from build123d import *

# Parameters (mm, degrees)
SALIENTE_EXTRUIR3_DEPTH = 0.02
SALIENTE_EXTRUIR5_START = -2
SALIENTE_EXTRUIR5_DEPTH = 2
CROQUIS4_R              = 0.025
SALIENTE_EXTRUIR6_DEPTH = 30
SALIENTE_EXTRUIR7_START = 0.01
CROQUIS4_2_R            = 0.025
SALIENTE_EXTRUIR7_DEPTH = 0.01


with BuildPart() as part:
    # Croquis1 → Saliente-Extruir3 (new body)
    with BuildSketch(Plane.XY):
        with BuildLine():
            Line((-0.821642524, 0), (-1.5, 0))
            ThreePointArc((-1.5, 0), (-1.803592236, -0.268799536), (-2.059736596, -0.583142508))
            Line((-2.059736596, -0.583142508), (-0.821642524, -0.583142508))
            Line((-0.821642524, -0.583142508), (0.708153247, -0.583142508))
            ThreePointArc((0.708153247, -0.583142508), (0.792032388, -0.667021649), (0.708153247, -0.75090079))
            Line((0.708153247, -0.75090079), (-0.821642524, -0.75090079))
            ThreePointArc((-0.821642524, -0.75090079), (-1.266985163, -1.19624343), (-0.821642524, -1.641586069))
            Line((-0.821642524, -1.641586069), (0.708153247, -1.641586069))
            ThreePointArc((0.708153247, -1.641586069), (0.788738621, -1.722171443), (0.708153247, -1.802756818))
            Line((0.708153247, -1.802756818), (-0.821642524, -1.802756818))
            ThreePointArc((-0.821642524, -1.802756818), (-1.277929981, -2.259044275), (-0.821642524, -2.715331733))
            Line((-0.821642524, -2.715331733), (0.708153247, -2.715331733))
            ThreePointArc((0.708153247, -2.715331733), (0.785471646, -2.792650132), (0.708153247, -2.869968532))
            Line((0.708153247, -2.869968532), (-0.821642524, -2.869968532))
            ThreePointArc((-0.821642524, -2.869968532), (-1.276795627, -3.325121635), (-0.821642524, -3.780274738))
            Line((-0.821642524, -3.780274738), (0.764779262, -3.780274738))
            Line((0.764779262, -3.780274738), (0.764779262, -4))
            Line((0.764779262, -4), (1.5, -4))
            ThreePointArc((1.5, -4), (1.806680275, -3.727977542), (2.064782817, -3.409493497))
            Line((2.064782817, -3.409493497), (-0.821642524, -3.409493497))
            ThreePointArc((-0.821642524, -3.409493497), (-0.907365435, -3.323770586), (-0.821642524, -3.238047675))
            Line((-0.821642524, -3.238047675), (0.708153247, -3.238047675))
            ThreePointArc((0.708153247, -3.238047675), (1.160084738, -2.786116183), (0.708153247, -2.334184692))
            Line((0.708153247, -2.334184692), (-0.821642524, -2.334184692))
            ThreePointArc((-0.821642524, -2.334184692), (-0.894604957, -2.261222258), (-0.821642524, -2.188259825))
            Line((-0.821642524, -2.188259825), (0.708153247, -2.188259825))
            ThreePointArc((0.708153247, -2.188259825), (1.169203972, -1.727209099), (0.708153247, -1.266158374))
            Line((0.708153247, -1.266158374), (-0.821642524, -1.266158374))
            ThreePointArc((-0.821642524, -1.266158374), (-0.890869473, -1.196931424), (-0.821642524, -1.127704475))
            Line((-0.821642524, -1.127704475), (0.708153247, -1.127704475))
            ThreePointArc((0.708153247, -1.127704475), (1.166166615, -0.669691107), (0.708153247, -0.211677738))
            Line((0.708153247, -0.211677738), (-0.821642524, -0.211677738))
            Line((-0.821642524, -0.211677738), (-0.821642524, 0))
        make_face()
    extrude(amount=SALIENTE_EXTRUIR3_DEPTH)

    # Croquis1_5 → Saliente-Extruir5 (add)
    with BuildSketch(Plane.XY.offset(SALIENTE_EXTRUIR5_START)):
        with BuildLine():
            Line((-0.821642524, -0.583142508), (-2.059736596, -0.583142508))
            ThreePointArc((-2.059736596, -0.583142508), (-2.467115713, -2.404153511), (-1.5, -4))
            Line((-1.5, -4), (0.764779262, -4))
            Line((0.764779262, -4), (0.764779262, -3.780274738))
            Line((0.764779262, -3.780274738), (-0.821642524, -3.780274738))
            ThreePointArc((-0.821642524, -3.780274738), (-1.276795627, -3.325121635), (-0.821642524, -2.869968532))
            Line((-0.821642524, -2.869968532), (0.708153247, -2.869968532))
            ThreePointArc((0.708153247, -2.869968532), (0.785471646, -2.792650132), (0.708153247, -2.715331733))
            Line((0.708153247, -2.715331733), (-0.821642524, -2.715331733))
            ThreePointArc((-0.821642524, -2.715331733), (-1.277929981, -2.259044275), (-0.821642524, -1.802756818))
            Line((-0.821642524, -1.802756818), (0.708153247, -1.802756818))
            ThreePointArc((0.708153247, -1.802756818), (0.788738621, -1.722171443), (0.708153247, -1.641586069))
            Line((0.708153247, -1.641586069), (-0.821642524, -1.641586069))
            ThreePointArc((-0.821642524, -1.641586069), (-1.266985163, -1.19624343), (-0.821642524, -0.75090079))
            Line((-0.821642524, -0.75090079), (0.708153247, -0.75090079))
            ThreePointArc((0.708153247, -0.75090079), (0.792032388, -0.667021649), (0.708153247, -0.583142508))
            Line((0.708153247, -0.583142508), (-0.821642524, -0.583142508))
        make_face()
        with BuildLine():
            Line((1.5, 0), (-0.821642524, 0))
            Line((-0.821642524, 0), (-0.821642524, -0.211677738))
            Line((-0.821642524, -0.211677738), (0.708153247, -0.211677738))
            ThreePointArc((0.708153247, -0.211677738), (1.166166615, -0.669691107), (0.708153247, -1.127704475))
            Line((0.708153247, -1.127704475), (-0.821642524, -1.127704475))
            ThreePointArc((-0.821642524, -1.127704475), (-0.890869473, -1.196931424), (-0.821642524, -1.266158374))
            Line((-0.821642524, -1.266158374), (0.708153247, -1.266158374))
            ThreePointArc((0.708153247, -1.266158374), (1.169203972, -1.727209099), (0.708153247, -2.188259825))
            Line((0.708153247, -2.188259825), (-0.821642524, -2.188259825))
            ThreePointArc((-0.821642524, -2.188259825), (-0.894604957, -2.261222258), (-0.821642524, -2.334184692))
            Line((-0.821642524, -2.334184692), (0.708153247, -2.334184692))
            ThreePointArc((0.708153247, -2.334184692), (1.160084738, -2.786116183), (0.708153247, -3.238047675))
            Line((0.708153247, -3.238047675), (-0.821642524, -3.238047675))
            ThreePointArc((-0.821642524, -3.238047675), (-0.907365435, -3.323770586), (-0.821642524, -3.409493497))
            Line((-0.821642524, -3.409493497), (2.064782817, -3.409493497))
            ThreePointArc((2.064782817, -3.409493497), (2.466390198, -1.591442305), (1.5, 0))
        make_face()
        with BuildLine():
            Line((-0.821642524, 0), (-1.5, 0))
            ThreePointArc((-1.5, 0), (-1.803592236, -0.268799536), (-2.059736596, -0.583142508))
            Line((-2.059736596, -0.583142508), (-0.821642524, -0.583142508))
            Line((-0.821642524, -0.583142508), (0.708153247, -0.583142508))
            ThreePointArc((0.708153247, -0.583142508), (0.792032388, -0.667021649), (0.708153247, -0.75090079))
            Line((0.708153247, -0.75090079), (-0.821642524, -0.75090079))
            ThreePointArc((-0.821642524, -0.75090079), (-1.266985163, -1.19624343), (-0.821642524, -1.641586069))
            Line((-0.821642524, -1.641586069), (0.708153247, -1.641586069))
            ThreePointArc((0.708153247, -1.641586069), (0.788738621, -1.722171443), (0.708153247, -1.802756818))
            Line((0.708153247, -1.802756818), (-0.821642524, -1.802756818))
            ThreePointArc((-0.821642524, -1.802756818), (-1.277929981, -2.259044275), (-0.821642524, -2.715331733))
            Line((-0.821642524, -2.715331733), (0.708153247, -2.715331733))
            ThreePointArc((0.708153247, -2.715331733), (0.785471646, -2.792650132), (0.708153247, -2.869968532))
            Line((0.708153247, -2.869968532), (-0.821642524, -2.869968532))
            ThreePointArc((-0.821642524, -2.869968532), (-1.276795627, -3.325121635), (-0.821642524, -3.780274738))
            Line((-0.821642524, -3.780274738), (0.764779262, -3.780274738))
            Line((0.764779262, -3.780274738), (0.764779262, -4))
            Line((0.764779262, -4), (1.5, -4))
            ThreePointArc((1.5, -4), (1.806680275, -3.727977542), (2.064782817, -3.409493497))
            Line((2.064782817, -3.409493497), (-0.821642524, -3.409493497))
            ThreePointArc((-0.821642524, -3.409493497), (-0.907365435, -3.323770586), (-0.821642524, -3.238047675))
            Line((-0.821642524, -3.238047675), (0.708153247, -3.238047675))
            ThreePointArc((0.708153247, -3.238047675), (1.160084738, -2.786116183), (0.708153247, -2.334184692))
            Line((0.708153247, -2.334184692), (-0.821642524, -2.334184692))
            ThreePointArc((-0.821642524, -2.334184692), (-0.894604957, -2.261222258), (-0.821642524, -2.188259825))
            Line((-0.821642524, -2.188259825), (0.708153247, -2.188259825))
            ThreePointArc((0.708153247, -2.188259825), (1.169203972, -1.727209099), (0.708153247, -1.266158374))
            Line((0.708153247, -1.266158374), (-0.821642524, -1.266158374))
            ThreePointArc((-0.821642524, -1.266158374), (-0.890869473, -1.196931424), (-0.821642524, -1.127704475))
            Line((-0.821642524, -1.127704475), (0.708153247, -1.127704475))
            ThreePointArc((0.708153247, -1.127704475), (1.166166615, -0.669691107), (0.708153247, -0.211677738))
            Line((0.708153247, -0.211677738), (-0.821642524, -0.211677738))
            Line((-0.821642524, -0.211677738), (-0.821642524, 0))
        make_face()
    extrude(amount=SALIENTE_EXTRUIR5_DEPTH)

    # Croquis4 → Saliente-Extruir6 (add)
    with BuildSketch(Plane.XY):
        with Locations((1.8, -2)):
            Circle(CROQUIS4_R)
        with Locations((-1.8, -2)):
            Circle(CROQUIS4_R)
    extrude(amount=-SALIENTE_EXTRUIR6_DEPTH)

    # Croquis4_2 → Saliente-Extruir7 (add)
    with BuildSketch(Plane.XY.offset(SALIENTE_EXTRUIR7_START)):
        with Locations((1.8, -2)):
            Circle(CROQUIS4_2_R)
        with Locations((-1.8, -2)):
            Circle(CROQUIS4_2_R)
    extrude(amount=-SALIENTE_EXTRUIR7_DEPTH)


solid = part.part
Input: part model. Units: mm. Frame: model coordinates. A direction names the side the tool comes from. Give positions to 0.01 mm unless a question says otherwise; leave off trailing zeros. Order: outer loops, then holes, each group sorted by start corner. A loop starts at its lowest first (then second) coordinate and runs counter-clockwise, first axis right, second up. Notation, with made-up numbers: M 33.5,-27 L 57.5,-27 A19 ccw 57.5,-7 Z; hole C 62,14 d2. An arc over 180 degrees is marked long. Answer as a JSON object with one key per item and string values.
1. Pull-direction query (Y, two-part tool) for faces 3 (the flat face through (0, -4, -1)), 4 (the flat face through (0, -2, -2)), 5 (the flat face through (2, -2, 0)), 6 (the flat face through (0, 0, -1)); classes: +Y half, -Y half, draft (parallel to the pull), parting line (faces both ways), or undercut.
Result sheet:
{"face 3": "-Y half", "face 4": "draft", "face 5": "undercut", "face 6": "+Y half"}
2. Reachability of faces 1 (the flat face through (0, -2, 0.02)), 2 (the flat face through (-2, -2, 0)) from +Z, -Z, +X, -X, +Y, -Y: full face, straight path, thin tool, end or side. Return the list, or none.
Result sheet:
{"face 1": "+Z, +X, -X, +Y, -Y", "face 2": "+Z, -X"}
3. First-contact query: P1, Ø3, axis at x = 0.5, z = -8, coming from the +Y side (3 decimals). Flat tip, straight axial feed; report the tip coordinate or a pass-through.
Result sheet:
{"P1": "y = -1.975"}
4. Ray query, line 1 (Z direction, x = 0.8, y = -2.3). Return the intervals inside material, ascending. Write a range as [from, to].
Result sheet:
{"line 1": "[-2, 0]"}
5. Cut plane A-A, the plane z = -20. Output: boundary loops of the cut face in (x, y) (3 decimals), and give its area (3 significant figures).
Result sheet:
{"outline": "C -1.8,-2 d0.05; C 1.8,-2 d0.05", "area": "0.00393 mm²"}
